Verification items for the finished model (mm, model axes). Face numbers are marked on the shaded views. A direction names the side the tool comes from. Round coordinates to 2 decimals unless told otherwise and drop trailing zeros. Order: outer loops, then holes, each group sorted by start corner. A loop starts at its lowest first (then second) coordinate and runs counter-clockwise, first axis right, second up. Notation, with made-up numbers: M 74,2 L 122,2 A32 ccw 122,37 Z; hole C 80,-20.5 d1. An arc over 180 degrees is marked long. Use one line per item in the form item = value. Start each with the question number.
Item 1: Cross-section at C-C on x = -7.5. Enter the section's corners in (y, z), then the cut area to 3 significant figures.
Item 2: Go/stop test with a flat-tipped pin: pin 1 Ø3.5 at (x, z) = (-5, 0.5) entering from -Y. Record where the tip stops, or that it passes through.
Item 3: Tool access check on the marked faces 1 and 2. Record the directions out of +Z, -Z, +X, -X, +Y, -Y that give a thin tool (end or side, any length) a straight path to the whole face; none if there is none.
Item 4: Thickness scan on probe 1 along Y at (x, z) = (-6.25, 4); probe 2 along Z at (x, y) = (-6.5, -0.15); probe 3 along Z at (x, y) = (-3.25, -0.15). Record the ranges inside material, lowest first. Write a range as [from, to].
Item 5: Cross-section at B-B on y = -0.6. Enter the section's corners in (x, z), then the cut area to 3 significant figures.
Item 6: Cross-section at A-A on z = 5.25. Enter the section's corners in (x, y).
from build123d import *

# Parameters (mm, degrees)
BASE_FLANGE1_DEPTH           = 0.2
EDGE_FLANGE1_STRIP_W         = 1.2
EDGE_FLANGE1_STRIP_H         = 0.2
EDGE_FLANGE1_STRIP_CUT_DEPTH = 11.5
EDGE_FLANGE1_DEPTH           = 11.5
F_1_7_1_7_DIAMETER_HOLE1_D   = 1.7


# Sheet-metal steps are written as plain solids
with BuildPart() as part:
    # Sketch1 → Base-Flange1 (new body)
    with BuildSketch(Plane(origin=(0, 0, 0), x_dir=(1, 0, 0), z_dir=(0, 1, 0))):
        Polygon((-4.873652989, 5.318528304), (-8.5, 1.692181293), (-8.5, -4.967910087), (-6.446655485, -7.021254602), (-0.949979928, -7.021254602), (3.258074995, -2.813199679), align=None)
    extrude(amount=-BASE_FLANGE1_DEPTH)

    # Edge-Flange1 strip (across the edge) → Edge-Flange1 strip cut (cut)
    with BuildSketch(Plane(origin=(-4.873652989, -0.2, -5.318528304), x_dir=(-0.7071067811865558, -3.4914813388431334e-15, 0.7071067811865392), z_dir=(0.7071067811865392, 0, 0.7071067811865558))):
        with Locations((-0.4, -0.1)):
            Rectangle(EDGE_FLANGE1_STRIP_W, EDGE_FLANGE1_STRIP_H)
    extrude(amount=EDGE_FLANGE1_STRIP_CUT_DEPTH, mode=Mode.SUBTRACT)

    # Edge-Flange1 section (across the edge) → Edge-Flange1 (add)
    with BuildSketch(Plane(origin=(-4.873652989, -0.2, -5.318528304), x_dir=(-0.7071067811865558, -3.4914813388431334e-15, 0.7071067811865392), z_dir=(0.7071067811865392, 0, 0.7071067811865558))):
        with BuildLine():
            Line((-0.2, 0.2), (-0.2, 0.8))
            Line((-0.2, 0.8), (0, 0.8))
            Line((0, 0.8), (0, 0.2))
            ThreePointArc((0, 0.2), (0.058578644, 0.058578644), (0.2, 0))
            Line((0.2, 0), (0.2, -0.2))
            ThreePointArc((0.2, -0.2), (-0.082842712, -0.082842712), (-0.2, 0.2))
        make_face()
    extrude(amount=EDGE_FLANGE1_DEPTH)

    # Ø1.7 (1.7) Diameter Hole1 (through all)
    with Locations(Plane(origin=(0, 0, 0), x_dir=(1, 0, 0), z_dir=(0, 1, 0))):
        with Locations((-6.5, -1.311055838), (-3, -4.811055838)):
            Hole(F_1_7_1_7_DIAMETER_HOLE1_D / 2)


solid = part.part
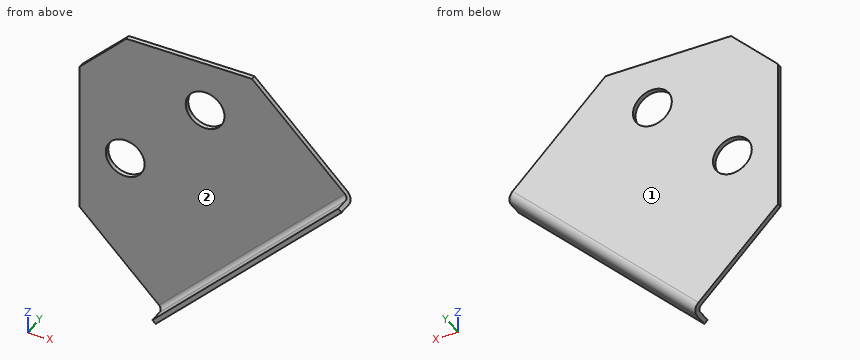
Output values:
q1.outline = M -0.2,-2.69 L 0,-2.69 L 0,5.97 L -0.2,5.97 Z
q1.area = 1.73 mm2
q2.pin_1 = -0.2
q3.face_1 = +Z, -Z, +X, -X, +Y
q3.face_2 = +Z, -X, -Y
q4.probe_1 = [-0.2, 0]
q4.probe_2 = [-3.69, 0.46], [2.16, 6.97]
q4.probe_3 = [-3.85, 4], [5.62, 7.02]
q5.outline = M -4.87,-5.32 L -4.73,-5.46 L 3.4,2.67 L 3.26,2.81 Z
q5.area = 2.30 mm2
q6.outline = M -8.22,-0.2 L -3.73,-0.2 L -3.73,0 L -8.22,0 Z; M -2.27,-0.2 L 0.82,-0.2 L 0.82,0 L -2.27,0 Z
